from build123d import *

# Parameters (mm, degrees)
SKIZZE1_W                       = 350
SKIZZE1_H                       = 250
AUFSATZ_LINEAR_AUSTRAGEN1_DEPTH = 10
VERRUNDUNG1_R                   = 5
SKIZZE3_W                       = 50
SKIZZE3_H                       = 30
SCHNITT_LINEAR_AUSTRAGEN1_DEPTH = 216.290501416


with BuildPart() as part:
    # Skizze1 → Aufsatz-Linear austragen1 (new body)
    with BuildSketch(Plane.XY):
        Rectangle(SKIZZE1_W, SKIZZE1_H)
    extrude(amount=AUFSATZ_LINEAR_AUSTRAGEN1_DEPTH)

    # Verrundung1
    verrundung1_edges = [part.edges().sort_by_distance(p)[0] for p in [
        (-175, 125, 5),
        (175, 125, 5),
        (175, -125, 5),
        (-175, -125, 5),
    ]]
    fillet(verrundung1_edges, radius=VERRUNDUNG1_R)

    # Skizze3 → Schnitt-Linear austragen1 (cut, through all)
    with BuildSketch(Plane.XY.offset(10)):
        Rectangle(SKIZZE3_W, SKIZZE3_H)
    extrude(amount=-SCHNITT_LINEAR_AUSTRAGEN1_DEPTH, mode=Mode.SUBTRACT)


solid = part.part
The model under review builds one solid part; all positions refer to its coordinate system, in mm. A direction names the side the tool comes from. Give positions to 0.01 mm unless a question says otherwise; leave off trailing zeros. Loops run counter-clockwise (first coordinate to the right, second up) from the corner with the lowest first, then second, coordinate; pieces in that order, holes last. Notation, with made-up numbers: (84, 52.25) -> (123, 52.25) arc R13 cw to (123, 73.25) -> close; hole circle Ø4 at (-16.5, 86). An arc over 180 degrees is marked (long way). Answer as a JSON object with one key per item and string values. Group by question number.
Q1. Insertion check: pin 1 (4 mm diameter, centred on x = 112.5, y = -42.5, fed in from -Z). The pin has a flat end and moves straight along its axis. Give the tip position at first contact, or say it passes through.
Q2. Take a section at A-A (z = 8.5). Write out the cut boundary in (x, y), plus the area to 3 significant figures.
Q3. Wall thickness on line 1 along Y through (x, z) = (-8, 2.25): over which ranges is the line inside the solid? List them lowest first.
Q4. Take a section at B-B (y = 11). Write out the cut boundary in (x, z).
Q5. Tool access review of faces 1 (the flat face through (0, -15, 5)), 2 (the flat face through (175, -2, 5)): name each direction out of +Z, -Z, +X, -X, +Y, -Y from which nothing blocks a thin tool from reaching the whole face with its end or side.
Q6. Take a section at C-C (x = 5). Write out the cut boundary in (y, z).
Q7. Draft analysis for pull direction X (two halves, no side actions). For faces 3 (the flat face through (-2, -125, 5)), 4 (the flat face through (-175, -2, 5)), 5 (the flat face through (25, 0, 5)), 6 (the flat face through (0, 15, 5)), state which applies: pulls with the +X half, pulls with the -X half, needs draft (parallel to the pull), parting line crosses it, or undercut.
Answer below:
{
 "1": {"pin 1": "stops at z = 0"},
 "2": {"outline": "(-175, -120) arc R5 ccw to (-170, -125) -> (170, -125) arc R5 ccw to (175, -120) -> (175, 120) arc R5 ccw to (170, 125) -> (-170, 125) arc R5 ccw to (-175, 120) -> close; hole (-25, -15) -> (25, -15) -> (25, 15) -> (-25, 15) -> close", "area": "86,000 mm2"},
 "3": {"line 1": "y = -125 to -15, 15 to 125"},
 "4": {"outline": "(-175, 0) -> (-25, 0) -> (-25, 10) -> (-175, 10) -> close; (25, 0) -> (175, 0) -> (175, 10) -> (25, 10) -> close"},
 "5": {"face 1": "+Z, -Z", "face 2": "+Z, -Z, +X, +Y, -Y"},
 "6": {"outline": "(-125, 0) -> (-15, 0) -> (-15, 10) -> (-125, 10) -> close; (15, 0) -> (125, 0) -> (125, 10) -> (15, 10) -> close"},
 "7": {"face 3": "needs draft", "face 4": "pulls with the -X half", "face 5": "undercut", "face 6": "undercut"}
}
